Model file for the job. Use its own axes, mm. A direction names the side the tool comes from. Round coordinates to 2 decimals unless told otherwise and drop trailing zeros. Order: outer loops, then holes, each group sorted by start corner. A loop starts at its lowest first (then second) coordinate and runs counter-clockwise, first axis right, second up. Notation, with made-up numbers: (64, 13.25) - (92, 13.25) arc R26 cw to (92, 34.25) - close; hole circle Ø1 at (72.5, 79.25). An arc over 180 degrees is marked (long way). Answer as CSV lines item,"result". Start each with the question number.
1. Band-saw the part on D-D on x = 1. List the corners of the cut face in (y, z).
2. Pull direction X, two halves, no side cores. Call faces 1 (the face through (10, -13, 0)), 2 (the face through (7, -14, -0.508)), 3 (the face through (1.786, -9.971, 2.068)), 4 (the face through (0, -13, 2)): released by +X, released by -X, zero draft, split by the parting line, or undercut.
3. 3-axis set-ups, long thin cutter, end or side, ignore diameter. For faces 5 (the face through (-1, -13, 0)), 6 (the face through (9.525, -13, 2)), 7 (the face through (4.7, -15.3, -6.35)): which of +Z, -Z, +X, -X, +Y, -Y reach the whole face in a straight line?
4. Band-saw the part on B-B on x = 3.75. List the corners of the cut face in (y, z), then the cut area to 3 significant figures.
5. Wall check: line 1 along X through (y, z) = (-0.75, 2.75) (3 decimals); line 2 along Y through (x, z) = (3.75, -4.75); line 3 along Z through (x, y) = (-0.25, -11.75). Give the ranges that are in metal, low to high. Write a range as [from, to].
6. Pin check, flat tips, straight feed: pin 1 Ø1.7 at (x, y) = (10, -11.5) entering from +Z; pin 2 Ø0.5 at (x, y) = (-1, -11.5) entering from +Z; pin 3 Ø1 at (y, z) = (-6.5, 2) entering from -X; pin 4 Ø2.5 at (x, y) = (3.5, -14.5) entering from +Z. Stop position of each tip, or through.
```python
from build123d import *

# Parameters (mm, degrees)
F0_W     = 9.525
F0_H     = 4.572
F1_DEPTH = 25.4
F2_R     = 4.0386
F3_DEPTH = 5.08
F4_R     = 2.2225
F5_DEPTH = 5.843


with BuildPart() as f1:
    # F0 (on Front) → F1 (new body)
    with BuildSketch(Plane.XZ):
        with Locations((4.7625, 2.286)):
            Rectangle(F0_W, F0_H)
        Polygon((9.525, 0), (0, 0), (-1.5875, 0), (-1.5875, -6.35), (11.1125, -6.35), (11.1125, 0), align=None)
    extrude(amount=F1_DEPTH)

    # F2 (on face) → F3 (cut)
    with BuildSketch(Plane.XY.offset(4.572)):
        with Locations((4.7625, -12.7)):
            Circle(F2_R)
    extrude(amount=-F3_DEPTH, mode=Mode.SUBTRACT)

    # F4 (on face) → F5 (cut, through all)
    with BuildSketch(Plane.XY.offset(-0.508)):
        with Locations((4.7625, -12.7)):
            Circle(F4_R)
    extrude(amount=-F5_DEPTH, mode=Mode.SUBTRACT)


solid = f1.part
```
Reply:
1,outline,"(-25.4, -6.35) - (0, -6.35) - (0, 4.57) - (-11.23, 4.57) - (-11.23, -0.51) - (-14.17, -0.51) - (-14.17, 4.57) - (-25.4, 4.57) - close"
2,face 1,"zero draft"
2,face 2,"undercut"
2,face 3,"undercut"
2,face 4,"released by -X"
3,face 5,"+Z, -X, +Y, -Y"
3,face 6,"+Z, +X, +Y, -Y"
3,face 7,"-Z, +X, -X, +Y, -Y"
4,outline,"(-25.4, -6.35) - (-14.68, -6.35) - (-14.68, -0.51) - (-16.61, -0.51) - (-16.61, 4.57) - (-25.4, 4.57) - close; (-10.72, -6.35) - (0, -6.35) - (0, 4.57) - (-8.79, 4.57) - (-8.79, -0.51) - (-10.72, -0.51) - close"
4,area,"215 mm2"
5,line 1,"x = [0, 9.525]"
5,line 2,"y = [-25.4, -14.68], [-10.72, 0]"
5,line 3,"z = [-6.35, 0]"
6,pin 1,"stops at z = 4.57"
6,pin 2,"stops at z = 0"
6,pin 3,"stops at x = 0"
6,pin 4,"stops at z = -0.51"
